from build123d import *

# Parameters (mm, degrees)
F1_DEPTH  = 15
F3_DEPTH  = 8
F4_R      = 1
F6_DEPTH  = 2
F8_DEPTH  = 2
F10_DEPTH = 2
F12_DEPTH = 2


# Not quite as in the source:
# - a feature names something its author has since deleted; it is built from what else it names


with BuildPart() as f1:
    # F0 (on Top) → F1 (new body)
    with BuildSketch(Plane.XY):
        with BuildLine():
            Line((-28.3214918106, 39.0464443552), (-46.1799150741, 20.1475579913))
            Line((-46.1799150741, 20.1475579913), (-24.1265251153, -0.6917001902))
            Line((-24.1265251153, -0.6917001902), (-40.4306314886, -17.9457124323))
            Line((-40.4306314886, -17.9457124323), (1.5834453516, -17.9457124323))
            ThreePointArc((1.5834453516, -17.9457124323), (28.9057292456, 7.2125327526), (-6.6504706629, 17.9457124323))
            Line((-6.6504706629, 17.9457124323), (-28.3214918106, 39.0464443552))
        make_face()
    extrude(amount=F1_DEPTH)

    # F2 (on face) → F3 (cut)
    with BuildSketch(Plane.XY.offset(15)):
        with BuildLine():
            Line((-2.5950646959, 16.9163886458), (3.7065453362, -15.5357513577))
            ThreePointArc((3.7065453362, -15.5357513577), (26.9474296129, 5.8151003686), (-2.5950646959, 16.9163886458))
        make_face()
        Polygon((-5.1901293918, 15.8294621167), (-34.8258907848, -15.5329307781), (0, -15.4121983796), align=None)
        Polygon((-28.8714991264, 35.28469053), (-43.1752689183, 20.1475579913), (-22.7079026012, 1.9694547007), (-8.9844264049, 16.4924847199), align=None)
    extrude(amount=-F3_DEPTH, mode=Mode.SUBTRACT)

    # F4
    f4_edges = [f1.edges().sort_by_distance(p)[0] for p in [
        (-37.250703, 29.597001, 0),
        (-35.15322, 9.727929, 0),
        (-32.278578, -9.318706, 0),
        (-19.423593, -17.945712, 0),
        (28.905729, 7.212533, 0),
        (-17.485981, 28.496078, 0),
        (-18.927963, 25.888588, 15),
        (-36.023384, 27.716124, 15),
        (-32.941586, 11.058506, 15),
        (-15.846165, 9.23097, 15),
        (-17.412945, -15.472565, 15),
        (-20.00801, 0.148266, 15),
        (-2.595065, 0.208632, 15),
        (0.55574, 0.690319, 15),
        (26.94743, 5.8151, 15),
        (28.905729, 7.212533, 15),
        (-19.423593, -17.945712, 15),
        (-32.278578, -9.318706, 15),
        (-35.15322, 9.727929, 15),
        (-37.250703, 29.597001, 15),
        (-17.485981, 28.496078, 15),
        (-6.650471, 17.945712, 7.5),
        (-28.321492, 39.046444, 7.5),
        (-46.179915, 20.147558, 7.5),
        (-40.430631, -17.945712, 7.5),
        (-24.126525, -0.6917, 7.5),
        (1.583445, -17.945712, 7.5),
    ]]
    fillet(f4_edges, radius=F4_R)

    # F5 (on face) → F6 (cut)
    with BuildSketch(Plane.XY.offset(7)):
        Polygon((-29.1725099087, -12.9052552501), (-3.2478775829, -12.3988948762), (-7.4992091395, 8.8786818087), align=None)
        Polygon((-23.3146349898, 6.744285012), (-14.0517026385, 16.1163697069), (-29.1725099087, 30.4047130048), (-38.2205257573, 20.8295438638), align=None)
        with BuildLine():
            Line((0, 14.7073501721), (6.1764790816, -13.333094822))
            ThreePointArc((6.1764790816, -13.333094822), (24.8870467759, 5.4887589231), (0, 14.7073501721))
        make_face()
    extrude(amount=-F6_DEPTH, mode=Mode.SUBTRACT)

    # F7 (on face) → F8 (cut)
    with BuildSketch(Plane.XY.offset(5)):
        with BuildLine():
            Line((3.6986530758, 12.4016236514), (9.2264488339, -9.847166948))
            ThreePointArc((9.2264488339, -9.847166948), (20.4226323137, 4.7456631043), (3.6986530758, 12.4016236514))
        make_face()
    extrude(amount=-F8_DEPTH, mode=Mode.SUBTRACT)

    # F9 (on face) → F10 (cut)
    with BuildSketch(Plane.XY.offset(5)):
        Polygon((-9.698738344, 2.2434238344), (-19.8120251298, -8.6724534631), (-7.6682440939, -8.4352609186), align=None)
    extrude(amount=-F10_DEPTH, mode=Mode.SUBTRACT)

    # F11 (on face) → F12 (cut)
    with BuildSketch(Plane.XY.offset(5)):
        Polygon((-33.7495236595, 20.8295438638), (-23.5399451314, 10.7388715832), (-18.9629313805, 15.3698198505), (-29.1725099087, 25.4604921311), align=None)
    extrude(amount=-F12_DEPTH, mode=Mode.SUBTRACT)


solid = f1.part
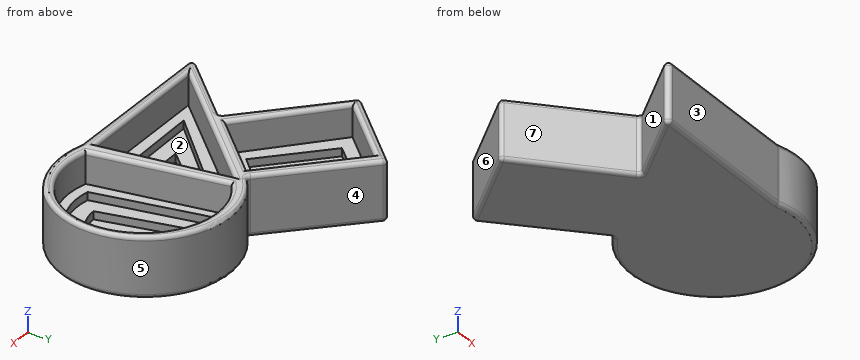
Here's how the part is built. I have some questions about the finished solid (model axes, mm). Face numbers are marked on the shaded views. A direction names the side the tool comes from. Coordinates: 2 decimals unless noted, no trailing zeros. Loops run counter-clockwise (first coordinate to the right, second up) from the corner with the lowest first, then second, coordinate; pieces in that order, holes last.
1. Imagine slicing it at A-A, the plane z = 8.75. Please give me the cut outline in (x, y).
2. If we mould it in two halves opening along Y, with no side actions, what happens to the marked faces 5, 6 and 7? For each: pulls with the +Y half, pulls with the -Y half, needs draft (parallel to the pull), parting line crosses it, or undercut.
3. I need wall thicknesses on L1, parallel to X at y = 9, z = 11.75; L2, parallel to X at y = 6, z = 11.25; L3, parallel to Y at x = -30, z = 12.75. Which ranges of each line are inside material? Lowest first, please.
4. For the marked faces 1, 2, 3 and 4, which set-ups out of +Z, -Z, +X, -X, +Y, -Y let a thin tool reach every point of the face, with its end or its side?
5. For P1, Ø13.5, axis at x = 15, y = 7.5, coming from the +Z side; P2, Ø8, axis at y = -8, z = 9.5, coming from the -X side; P3, Ø4, axis at x = -37.5, z = 13, coming from the +Y side, each with a flat end and sliding along its axis, tell me the tip position at first contact or that it passes through.
Taken from the geometry:
1. outline: (-45.49, 20.87) arc R1 ccw to (-45.45, 19.46) - (-24.85, 0) arc R1 cw to (-24.81, -1.42) - (-38.84, -16.26) arc R1 ccw to (-38.11, -17.95) - (1.43, -17.95) arc R1 cw to (1.73, -17.99) arc R21.38 ccw (long way) to (-5.97, 18.56) arc R1 cw to (-7.32, 18.6) - (-27.59, 38.34) arc R1 ccw to (-29.02, 38.31) - close; hole (-43.18, 20.15) - (-22.71, 1.97) - (-8.98, 16.49) - (-28.87, 35.28) - close; hole (-34.83, -15.53) - (0, -15.41) - (-5.19, 15.83) - close; hole (-2.6, 16.92) - (3.71, -15.54) arc R18.52 ccw (long way) to start
2. face 5: parting line crosses it
2. face 6: pulls with the +Y half
2. face 7: undercut
3. L1: x = -34.38 to -30.62, -16.06 to -11.64, -4.06 to -1.06, 26.03 to 28.41
3. L2: x = -31.21 to -27.25, -18.9 to -14.48, -3.56 to -0.48, 26.91 to 29.15
3. L3: y = -17.95 to -15.52, -10.43 to -6.91, 4.86 to 8.45, 34.09 to 37.27
4. face 1: +Z, -Z, -X
4. face 2: +Z
4. face 3: +Z, -Z, -X, -Y
4. face 4: +Z, -Z, +Y
5. P1: stops at z = 5
5. P2: stops at x = -34.81
5. P3: stops at y = 31.45
